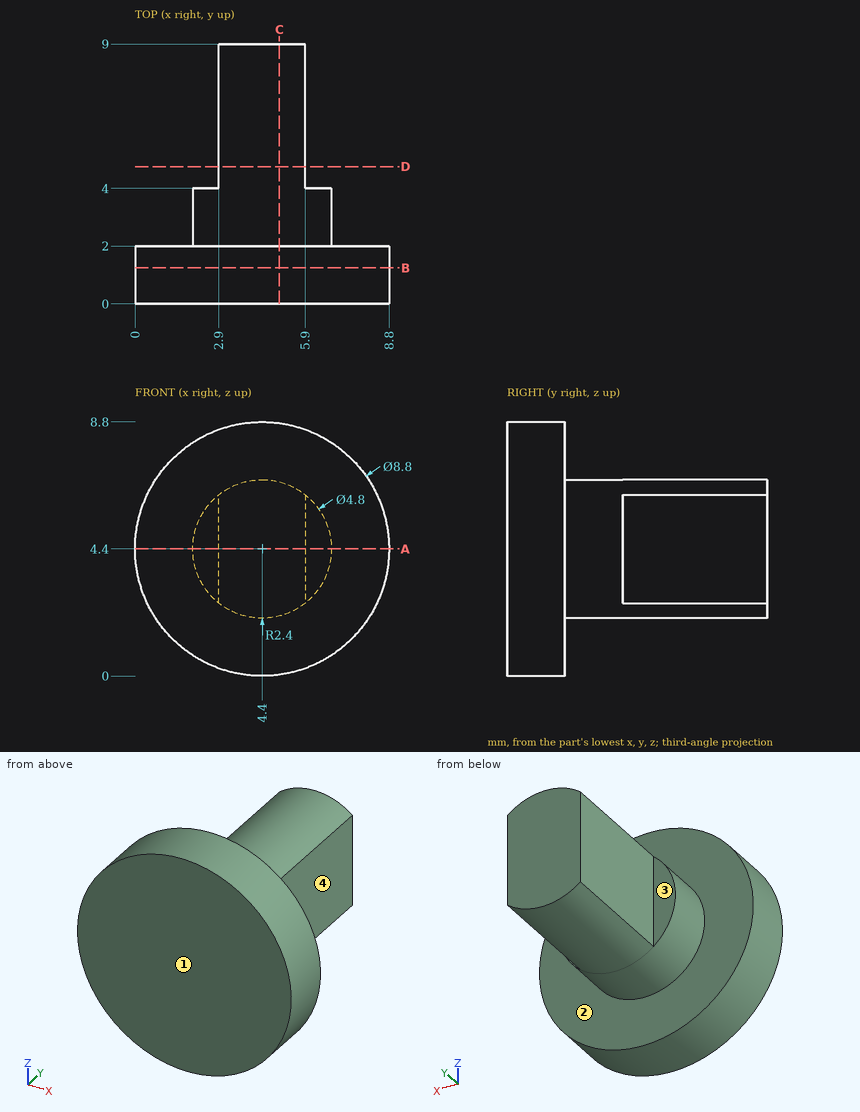
Source: three-view drawing plus pictorial views. Frame: mm from the lowest corner of the part. A direction names the side the tool comes from. Coordinates: 2 decimals unless noted, no trailing zeros. Write each loop counter-clockwise with the first axis right and the second up, starting at its lowest first coordinate (ties: lowest second). Pieces come first, ordered by that corner, then holes. Notation, with made-up numbers: (-37.5, 53) - (-17.5, 53) arc R15 cw to (-17.5, 68) - close; hole circle Ø4 at (43, 82). An arc over 180 degrees is marked (long way). Answer as a JSON object with one key per item and string values.
Q1. Section query D-D, the plane y = 4.75. Output: boundary loops of the cut face in (x, z).
Ans:
{"outline": "(2.9, 2.53) arc R2.4 ccw to (5.9, 2.53) - (5.9, 6.27) arc R2.4 ccw to (2.9, 6.27) - close"}
Q2. First-contact query: pin 1 Ø0.5 at (x, z) = (2.5, 4) entering from +Y; pin 2 Ø3 at (y, z) = (6.5, 3.5) entering from +X; pin 3 Ø1 at (x, z) = (7.5, 2.5) entering from +Y. Flat tips, straight axial feed; report the tip coordinate or a pass-through.
Ans:
{"pin 1": "stops at y = 4", "pin 2": "stops at x = 5.9", "pin 3": "stops at y = 2"}
Q3. Set-up query: the marked faces 1, 2, 3 and 4. Return all of +Z, -Z, +X, -X, +Y, -Y with unobstructed straight access to the full face (end or side cutting, diameter ignored); none if empty.
Ans:
{"face 1": "+Z, -Z, +X, -X, -Y", "face 2": "+Y", "face 3": "+Z, -Z, -X, +Y", "face 4": "+Z, -Z, +X, +Y"}
Q4. Section query C-C, the plane x = 5. Output: boundary loops of the cut face in (y, z).
Ans:
{"outline": "(0, 0.04) - (2, 0.04) - (2, 2.08) - (9, 2.08) - (9, 6.72) - (2, 6.72) - (2, 8.76) - (0, 8.76) - close"}
Q5. Section query B-B, the plane y = 1.25. Output: boundary loops of the cut face in (x, z).
Ans:
{"outline": "circle Ø8.8 at (4.4, 4.4)"}
Q6. Section query A-A, the plane z = 4.4. Output: boundary loops of the cut face in (x, y), plus the area to 3 significant figures.
Ans:
{"outline": "(0, 0) - (8.8, 0) - (8.8, 2) - (6.8, 2) - (6.8, 4) - (5.9, 4) - (5.9, 9) - (2.9, 9) - (2.9, 4) - (2, 4) - (2, 2) - (0, 2) - close", "area": "42.2 mm2"}
Q7. Material intervals for line 1 (Y direction, x = 7.5, z = 7.25); line 2 (X direction, y = 6.25, z = 3.25); line 3 (X direction, y = 0.5, z = 4.5), sorted ascending. Write a range as [from, to].
Ans:
{"line 1": "y = [0, 2]", "line 2": "x = [2.9, 5.9]", "line 3": "x = [0, 8.8]"}
